from build123d import *

# Parameters (mm, degrees)
SKETCH1_R           = 3
BOSS_EXTRUDE1_DEPTH = 2.8
SKETCH4_R           = 1.05
SKETCH5_R           = 0.5
CUT_EXTRUDE1_DEPTH  = 2.8


with BuildPart() as part:
    # Sketch1 → Boss-Extrude1 (new body)
    with BuildSketch(Plane(origin=(0, 0, 0), x_dir=(0, 0, -1), z_dir=(1, 0, 0))):
        Circle(SKETCH1_R)
    extrude(amount=BOSS_EXTRUDE1_DEPTH)

    # Sketch4 → Revolve1 (revolve)
    with BuildSketch(Plane.XY, mode=Mode.PRIVATE) as revolve1_sk:
        with Locations((1.4, 3)):
            Circle(SKETCH4_R)
    revolve(revolve1_sk.sketch.rotate(Axis((0, 0, 0), (1, 0, 0)), 180), axis=Axis((0, 0, 0), (1, 0, 0)))

    # Sketch5 → Cut-Extrude1 (cut)
    with BuildSketch(Plane(origin=(2.8, 0, 0), x_dir=(0, 0, -1), z_dir=(1, 0, 0))):
        Circle(SKETCH5_R)
    extrude(amount=-CUT_EXTRUDE1_DEPTH, mode=Mode.SUBTRACT)


solid = part.part
Read the model definition and answer for the solid it produces. Units are mm, in the model's axes. A direction names the side the tool comes from. Coordinates: 2 decimals unless noted, no trailing zeros. Loops run counter-clockwise (first coordinate to the right, second up) from the corner with the lowest first, then second, coordinate; pieces in that order, holes last. Notation, with made-up numbers: (14, -9.5) -> (37, -9.5) arc R18 ccw to (37, -3.5) -> close; hole circle Ø11 at (33.5, 79). An arc over 180 degrees is marked (long way). Write item = value, one per line. Start each with the question number.
1) The part is cut by section C-C, the plane x = 1.2. Determine the outline of the cut face in (y, z).
2) Given P1, Ø1.5, axis at x = 2.5, y = -0.5, coming from the +Z side, flat-ended and moving along its own axis, determine where the tip first touches the part or whether it passes through.
3) For faces 1 (the face through (2.8, 0, -1)), 2 (the face through (2.62, -1.15, -2.77)), 3 (the face through (0.2, 0.1, 3)), determine the directions among +Z, -Z, +X, -X, +Y, -Y from which every point of the face is accessible in a straight line to the end or side of a thin tool.
4) Find the intervals of material crossed by L1, parallel to X at y = -2, z = -3; L2, parallel to Z at x = 0.55, y = 1.25; L3, parallel to Z at x = 2.15, y = 1.75, in increasing order. Write a range as from..to.
5) The part is cut by section A-A, the plane z = 0. Determine the outline of the cut face in (x, y).
Result:
q1.outline = circle Ø8.06 at (0, 0); hole circle Ø1 at (0, 0)
q2.P1 = 3.97
q3.face_1 = +Z, -Z, +X, +Y, -Y
q3.face_2 = +X
q3.face_3 = -X
q4.L1 = 0.54..2.26
q4.L2 = -3.39..3.39
q4.L3 = -3.3..3.3
q5.outline = (0, -3) -> (0.35, -3) arc R1.05 ccw to (2.45, -3) -> (2.8, -3) -> (2.8, -0.5) -> (0, -0.5) -> close; (0, 0.5) -> (2.8, 0.5) -> (2.8, 3) -> (2.45, 3) arc R1.05 ccw to (0.35, 3) -> (0, 3) -> close
